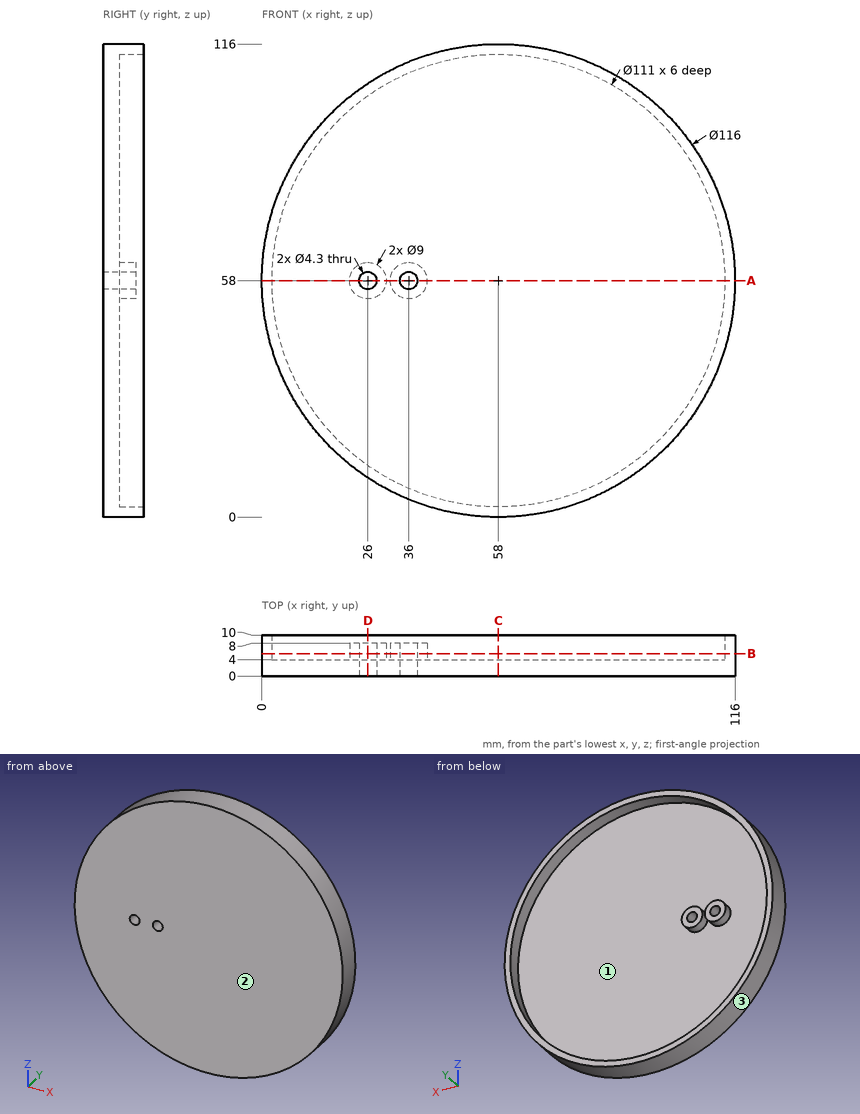
Verification items for this drawing (mm, ordinates from the low corner). Give positions to 0.01 mm unless a question says otherwise; leave off trailing zeros. Loops run counter-clockwise (first coordinate to the right, second up) from the corner with the lowest first, then second, coordinate; pieces in that order, holes last. Notation, with made-up numbers: M 24.5,24 L 65.5,24 A18 ccw 65.5,53 Z; hole C 22.5,-38 d1. An arc over 180 degrees is marked long. Answer as a JSON object with one key per item and string values. Group by question number.
Item 1: Sectioned sample at D-D on x = 26. Record the boundary of the cut face in (y, z).
Item 2: Sectioned sample at A-A on z = 58. Record the boundary of the cut face in (x, y), plus the area to 3 significant figures.
Item 3: Sectioned sample at C-C on x = 58. Record the boundary of the cut face in (y, z).
Item 4: Gauge pin test, flat ends, axial feed: pin 1 (3 mm diameter, centred on x = 70.5, y = 7, fed in from +Z); pin 2 (3 mm diameter, centred on y = 3.5, z = 50, fed in from +X); pin 3 (4 mm diameter, centred on x = 17.5, y = 5, fed in from -Z). Record the tip position at first contact, or that the pin passes through.
Item 5: Sectioned sample at B-B on y = 5.5. Record the boundary of the cut face in (x, z), plus the area to 3 significant figures.
Item 6: Material ranges on L1, parallel to X at y = 6.1, z = 58; L2, parallel to X at y = 2, z = 58; L3, parallel to Y at x = 32, z = 41, recorded low to high.
Item 7: Mould release check, pull along X, two halves, no side actions. Record for the marked faces 1, 2 and 3: pulls with the +X half, pulls with the -X half, needs draft (parallel to the pull), parting line crosses it, or undercut.
Findings below:
{
 "1": {"outline": "M 0,9.63 L 10,9.63 L 10,12.65 L 4,12.65 L 4,53.5 L 8,53.5 L 8,55.85 L 0,55.85 Z; M 0,60.15 L 8,60.15 L 8,62.5 L 4,62.5 L 4,103.35 L 10,103.35 L 10,106.37 L 0,106.37 Z"},
 "2": {"outline": "M 0,0 L 23.85,0 L 23.85,8 L 21.5,8 L 21.5,4 L 2.5,4 L 2.5,10 L 0,10 Z; M 28.15,0 L 33.85,0 L 33.85,8 L 31.5,8 L 31.5,4 L 30.5,4 L 30.5,8 L 28.15,8 Z; M 38.15,0 L 116,0 L 116,10 L 113.5,10 L 113.5,4 L 40.5,4 L 40.5,8 L 38.15,8 Z", "area": "497 mm2"},
 "3": {"outline": "M 0,0 L 10,0 L 10,2.5 L 4,2.5 L 4,113.5 L 10,113.5 L 10,116 L 0,116 Z"},
 "4": {"pin 1": "z = 114.95", "pin 2": "x = 115.63", "pin 3": "z = 14.62"},
 "5": {"outline": "C 58,58 d116; C 26,58 d9; C 36,58 d9; hole C 58,58 d111; hole C 26,58 d4.3; hole C 36,58 d4.3", "area": "990 mm2"},
 "6": {"L1": "0 to 2.5, 21.5 to 23.85, 28.15 to 30.5, 31.5 to 33.85, 38.15 to 40.5, 113.5 to 116", "L2": "0 to 23.85, 28.15 to 33.85, 38.15 to 116", "L3": "0 to 4"},
 "7": {"face 1": "undercut", "face 2": "needs draft", "face 3": "parting line crosses it"}
}
